```python
from build123d import *

# Parameters (mm, degrees)
SKETCH_R          = 12.236691
PAD_DEPTH         = 100
PAD001_DEPTH      = 10
SKETCH002_R       = 9.967721
PAD002_DEPTH      = 31
PAD002_DEPTH_BACK = -10
SKETCH003_R       = 2.654836
PAD003_DEPTH      = 5
SKETCH004_R       = 10.291555
SKETCH004_R_2     = 5.760448
POCKET_DEPTH      = 110.001
SKETCH005_R       = 8.252369
POCKET001_DEPTH   = 56


with BuildPart() as part:
    # Sketch → Pad (new body)
    with BuildSketch(Plane.XY):
        Circle(SKETCH_R)
    extrude(amount=PAD_DEPTH)

    # Sketch001 (on Face3 of Pad) → Pad001 (join)
    with BuildSketch(Plane.XY.offset(100)):
        with BuildLine():
            ThreePointArc((-20.361812, 3.080584), (0.000187, -20.593527), (20.361756, 3.080953))
            Line((11.095306, 64.322127), (20.361756, 3.080953))
            ThreePointArc((11.095306, 64.322127), (0.004574, 75.125929), (-11.095059, 64.33127))
            Line((-11.095059, 64.33127), (-20.361812, 3.080584))
        make_face()
    extrude(amount=PAD001_DEPTH)

    # Sketch002 (on DatumPlane) → Pad002 (join, two sides)
    with BuildSketch(Plane(origin=(0, -25, 50), x_dir=(-1, 0, 0), z_dir=(0, -0.707107, 0.707107))) as pad002_sk:
        Circle(SKETCH002_R)
    extrude(amount=-PAD002_DEPTH)
    extrude(pad002_sk.sketch, amount=-PAD002_DEPTH_BACK)

    # Sketch003 (on Face10 of Pad002) → Pad003 (join)
    with BuildSketch(Plane(origin=(0, -44.571068, 44.571068), x_dir=(1, 0, 0), z_dir=(0, -0.707107, 0.707107))):
        with BuildLine():
            ThreePointArc((4.5502, 30.252493), (0, 31.046218), (-4.5502, 30.252493))
            Line((-27.904433, 21.84908), (-4.5502, 30.252493))
            ThreePointArc((-27.904433, 21.84908), (-31.066679, 17.606865), (-27.904433, 13.36465))
            Line((-4.5502, 4.961238), (-27.904433, 13.36465))
            ThreePointArc((-4.5502, 4.961238), (0, 4.167512), (4.5502, 4.961238))
            Line((27.904433, 13.36465), (4.5502, 4.961238))
            ThreePointArc((27.904433, 13.36465), (31.066679, 17.606865), (27.904433, 21.84908))
            Line((4.5502, 30.252493), (27.904433, 21.84908))
        make_face()
        with Locations((-26.640049, 17.606865)):
            Circle(SKETCH003_R, mode=Mode.SUBTRACT)
        with Locations((26.640049, 17.606865)):
            Circle(SKETCH003_R, mode=Mode.SUBTRACT)
    extrude(amount=PAD003_DEPTH)

    # Sketch004 (on Face21 of Pad003) → Pocket (cut, through all)
    with BuildSketch(Plane.XY.offset(110)):
        Circle(SKETCH004_R)
        with Locations((0, 61.864815)):
            Circle(SKETCH004_R_2)
    extrude(amount=-POCKET_DEPTH, mode=Mode.SUBTRACT)

    # Sketch005 (on Face5 of Pocket) → Pocket001 (cut)
    with BuildSketch(Plane(origin=(0, -48.106602, 48.106602), x_dir=(1, 0, 0), z_dir=(0, -0.707107, 0.707107))):
        with Locations((0, 17.562706)):
            Circle(SKETCH005_R)
    extrude(amount=-POCKET001_DEPTH, mode=Mode.SUBTRACT)


solid = part.part
```
Build history of the part. All positions in model axes, mm. A direction names the side the tool comes from. Coordinates: 2 decimals unless noted, no trailing zeros. Order: outer loops, then holes, each group sorted by start corner. A loop starts at its lowest first (then second) coordinate and runs counter-clockwise, first axis right, second up.
Item 1: Saw through at A-A on y = -4. List the corners of the cut face in (x, z).
Filled in:
outline: (-20.2, 100) - (-11.56, 100) - (-11.56, 0) - (-9.48, 0) - (-9.48, 110) - (-20.2, 110) - close; (9.48, 0) - (11.56, 0) - (11.56, 100) - (20.2, 100) - (20.2, 110) - (9.48, 110) - close
Item 2: Saw through at C-C on x = 0. List the corners of the cut face in (y, z), then the cut area to 3 significant figures.
Filled in:
outline: (-45.16, 51.05) - (-41.62, 47.52) - (-39.12, 50.02) - (-12.24, 23.14) - (-12.24, 0) - (-10.29, 0) - (-10.29, 23.46) - (-41.52, 54.69) - close; (-29.85, 66.36) - (-10.29, 46.8) - (-10.29, 110) - (-20.59, 110) - (-20.59, 100) - (-12.24, 100) - (-12.24, 51.33) - (-25.02, 64.12) - (-22.62, 66.52) - (-26.15, 70.06) - close; (10.29, 0) - (12.24, 0) - (12.24, 100) - (56.1, 100) - (56.1, 110) - (10.29, 110) - close; (67.63, 100) - (75.13, 100) - (75.13, 110) - (67.63, 110) - close
area: 1,130 mm2
Item 3: Tool access for faces 1 (the cylindrical face through (0.065, -24.361, 68.267)), 2 (the cylindrical face through (31.066, -33.92, 58.708)), 3 (the cylindrical face through (-1.593, 12.133, 49.3)): list every direction of +Z, -Z, +X, -X, +Y, -Y with a clear straight run to the whole face (end or side of a thin tool).
Filled in:
face 1: +Z
face 2: +X
face 3: none
Item 4: Drill centre lines: L1, parallel to Y at x = 0, z = 107.5; L2, parallel to X at y = -31, z = 55.5; L3, parallel to Y at x = 0, z = 88.5. Where is each one in solid material? Low to high.
Filled in:
L1: y = -20.59 to -10.29, 10.29 to 56.1, 67.63 to 75.13
L2: x = -9.96 to -8.25, 8.25 to 9.96
L3: y = -12.24 to -10.29, 10.29 to 12.24
Item 5: Saw through at B-B on x = -17.5. List the corners of the cut face in (y, z).
Filled in:
outline: (-41.3, 54.91) - (-37.77, 51.37) - (-26.47, 62.67) - (-30.01, 66.2) - close; (-10.86, 100) - (22, 100) - (22, 110) - (-10.86, 110) - close
Item 6: Mould opens along Y. For faces 4 (the cylindrical face through (-1.789, -25.933, 39.378)), 5 (the flat face through (-16.39, -27.93, 64.69)), 6 (the cylindrical face through (-0.065, -43.367, 49.261)), 7 (the flat face through (0, 28, 100)) say: released by +Y, released by -Y, zero draft, split by the parting line, or undercut.
Filled in:
face 4: undercut
face 5: undercut
face 6: released by -Y
face 7: zero draft
Item 7: Saw through at D-D on z = 9.5. List the corners of the cut face in (x, y), then the cut area to 3 significant figures.
Filled in:
outline: circle Ø24.47 at (0, 0); hole circle Ø20.58 at (0, 0)
area: 138 mm2
Item 8: Drop flat-ended pins along their axis: pin 1 Ø12 at (x, z) = (-12.5, 92) entering from -Y; pin 2 Ø3 at (y, z) = (-7, 95) entering from +X; pin 3 Ø7 at (x, y) = (0, 61.86) entering from +Z; pin 4 Ø6 at (x, z) = (13, 80) entering from -Y. Give the stop position or say it passes through.
Filled in:
pin 1: stops at y = -10.37
pin 2: stops at x = 10.93
pin 3: passes through
pin 4: stops at y = -7.05
